Autodesk Inventor part; units mm, degrees
ref_plane "YZ Plane" through (0, 0, 0) normal (1, 0, 0) x (0, 1, 0)
ref_plane "XZ Plane" through (0, 0, 0) normal (0, 1, 0) x (-1, 0, 0)
ref_plane "XY Plane" through (0, 0, 0) normal (0, 0, 1) x (1, 0, 0)
sketch "Esquisse1" plane through (0, 0, 0) normal (0, 0, 1) x (1, 0, 0)
  line L0 (0, 0) -> (20, 0)
  line L1 (20, 0) -> (20, 20)
  line L2 (20, 20) -> (0, 20)
  line L3 (0, 20) -> (0, 0)
  circle A0 centre (10, 10) radius 2.15
  dimension "d0" = 20
  dimension "d1" = 20
  dimension "d2" = 4.3
extrude "Extrusion1" add sketch "Esquisse1" along normal blind 4
sketch "Esquisse2" plane through (0, 0, 4) normal (0, 0, 1) x (1, 0, 0)
  circle A0 centre (10, 10) radius 2.15
  line L0 (0, 20) -> (0, 0)
  circle A1 centre (10, 10) radius 2.15
  line L1 (0, 0) -> (20, 0)
  line L2 (20, 0) -> (20, 20)
  line L3 (20, 20) -> (0, 20)
  line L4 (0, 20) -> (0, 0)
  line L5 (13.4897, 12.0384) -> (13.5102, 7.997)
  line L6 (13.5102, 7.997) -> (10.0204, 5.9586)
  line L7 (10.0204, 5.9586) -> (6.5103, 7.9616)
  line L8 (6.5103, 7.9616) -> (6.4898, 12.003)
  line L9 (6.4898, 12.003) -> (6.4898, 20)
  line L10 (20, 20) -> (0, 20)
  line L11 (13.4897, 12.0384) -> (13.4897, 20)
  line L12 (6.4898, 20) -> (0, 20)
  line L13 (0, 0) -> (20, 0)
  line L14 (0, 0) -> (0, 20)
  line L15 (0, 0) -> (20, 0)
  line L16 (20, 0) -> (20, 20)
  line L17 (20, 20) -> (13.4897, 20)
  dimension "d5" = 7
  dimension "d6" = 0.29
extrude "Extrusion2" add sketch "Esquisse2" along normal blind 3.2 contours L3 L9 L8 L7 L6 L5 L11 L2 L1 L0
sketch "Esquisse3" plane through (0, 0, 7.2) normal (0, 0, 1) x (1, 0, 0)
  line L0 (6.4898, 20) -> (0, 20)
  line L1 (0, 20) -> (20, 20)
  line L2 (20, 20) -> (20, 0)
  line L3 (20, 0) -> (0, 0)
  line L4 (0, 0) -> (0, 20)
  circle A0 centre (10, 10) radius 2.15
  circle A1 centre (10, 10) radius 2.15
  point P0 (0, 0)
extrude "Extrusion4" add sketch "Esquisse3" along normal blind 4
sketch "Esquisse4" plane through (0, 0, 11.2) normal (0, 0, 1) x (1, 0, 0)
  line L0 (0, 20) -> (0, 0)
  line L1 (0, 10) -> (0, 0)
  line L2 (0, 0) -> (20, 0)
  line L3 (20, 0) -> (20, 10)
  line L4 (20, 0) -> (20, 20)
  line L5 (10, 10) -> (2.5, 10) construction
  line L6 (2.5, 10) -> (17.5, 10) construction
  arc A0 (2.5, 10) -> (17.5, 10) centre (10, 10) ccw
  arc A1 (17.5, 10) -> (2.5, 10) centre (10, 10) ccw
  line L7 (0, 10) -> (0, 20)
  line L8 (20, 20) -> (0, 20)
  line L9 (0, 20) -> (20, 20)
  line L10 (20, 20) -> (20, 10)
  line L11 (0, 10) -> (1.5, 10)
  line L12 (18.5, 10) -> (20, 10)
  arc A2 (18.5, 10) -> (1.5, 10) centre (10, 10) ccw
  dimension "d15" = 7.5
  dimension "d16" = 1
extrude "Extrusion5" add sketch "Esquisse4" along normal blind 20 contours L11 A2 L12 L3 L2 L0
sketch "Esquisse5" plane through (0, 0, 31.2) normal (0, 0, 1) x (1, 0, 0)
  circle A0 centre (10, 10) radius 7.5
  line L0 (0, 0) -> (20, 0)
  line L1 (20, 0) -> (20, 10)
  line L2 (20, 10) -> (18.5, 10)
  arc A1 (18.5, 10) -> (1.5, 10) centre (10, 10) ccw
  line L3 (1.5, 10) -> (0, 10)
  line L4 (0, 10) -> (0, 0)
  arc A2 (18.5, 10) -> (1.5, 10) centre (10, 10) ccw
  line L5 (6.0494, 17.5262) -> (6.0494, 16.3752)
  line L6 (13.9506, 16.3752) -> (13.9506, 17.5262)
  arc A3 (18.5, 10) -> (1.5, 10) centre (10, 10) ccw
  circle A4 centre (10, 10) radius 7.5
extrude "Extrusion6" add sketch "Esquisse5" along normal blind 78.5 contours A0 L6 A1 L2 L1 L0 L4 L3 L5
sketch "Esquisse6" plane through (0, 0, 109.7) normal (0, 0, 1) x (1, 0, 0)
  arc A0 (6.0494, 16.3752) -> (13.9506, 16.3752) centre (10, 10) ccw
  line L0 (0, 0) -> (20, 0)
  line L1 (11, 0.567) -> (11, 2.567)
  line L2 (9, 0.567) -> (9, 2.567)
  arc A1 (9, 2.567) -> (11, 2.567) centre (10, 10) ccw
  line L3 (9, 0.567) -> (11, 0.567)
  dimension "d23" = 2
  dimension "d24" = 2
extrude "Extrusion7" cut sketch "Esquisse6" against normal blind 90
sketch "Esquisse7" plane through (0, 0, 0) normal (-1, 0, 0) x (0, 0, 1)
  point P0 (0, 0)
sketch "Esquisse8" plane through (0, 0, 0) normal (-1, 0, 0) x (0, 0, 1)
  line L0 (109.7, 0) -> (109.7, 10)
  line L1 (0, 0) -> (109.7, 0)
  line L2 (109.7, 0) -> (109.7, 5)
  line L3 (109.7, 5) -> (0, 5)
  line L4 (0, 5) -> (0, 0)
extrude "Extrusion8" add sketch "Esquisse8" along normal blind 10
sketch "Esquisse9" plane through (20, 0, 0) normal (1, 0, 0) x (0, 0, -1)
  line L0 (-109.7, 0) -> (-109.7, 10)
  line L1 (0, 0) -> (-109.7, 0)
  line L2 (-109.7, 0) -> (-109.7, 5)
  line L3 (-109.7, 5) -> (0, 5)
  line L4 (0, 5) -> (0, 0)
extrude "Extrusion9" add sketch "Esquisse9" along normal blind 10
sketch "Esquisse10" plane through (20, 5, 109.7) normal (0, 1, 0) x (1, 0, 0)
  line L0 (10.0235, 93.2538) -> (5.0235, 93.2538) construction
  line L1 (0, 98.5) -> (0, 0) construction
  line L2 (5.0235, 93.2538) -> (5.0235, 8.1061) construction
  circle A0 centre (5.0235, 93.2538) radius 2.15
  circle A1 centre (5.0235, 53.2538) radius 2.15
  circle A2 centre (5.0235, 13.2538) radius 2.15
  circle A3 centre (-24.9765, 93.2538) radius 2.15
  circle A4 centre (-24.9765, 53.2538) radius 2.15
  circle A5 centre (-24.9765, 13.2538) radius 2.15
  point P0 (-20, 109.7)
  dimension "d31" = 5
  dimension "d32" = 4.3
  dimension "d35" = 40
  dimension "d38" = 30
extrude "Extrusion10" cut sketch "Esquisse10" against normal blind 10
sketch "Esquisse11" plane through (0, 0, 109.7) normal (0, 0, 1) x (1, 0, 0)
  line L0 (9, 0.567) -> (9, 2.567)
  arc A0 (6.0494, 16.3752) -> (9, 2.567) centre (10, 10) ccw
  line L1 (6.0494, 16.3752) -> (6.0494, 17.5262)
  arc A1 (6.0494, 17.5262) -> (1.5, 10) centre (10, 10) ccw
  line L2 (1.5, 10) -> (0, 10)
  line L3 (0, 10) -> (0, 5)
  line L4 (0, 5) -> (-10, 5)
  line L5 (-10, 0) -> (-10, 5)
  line L6 (30, 0) -> (-10, 0)
  line L7 (30, 5) -> (30, 0)
  line L8 (20, 5) -> (30, 5)
  line L9 (20, 5) -> (20, 10)
  line L10 (20, 10) -> (18.5, 10)
  arc A2 (18.5, 10) -> (13.9506, 17.5262) centre (10, 10) ccw
  line L11 (13.9506, 17.5262) -> (13.9506, 16.3752)
  arc A3 (11, 2.567) -> (13.9506, 16.3752) centre (10, 10) ccw
  line L12 (11, 2.567) -> (11, 0.567)
  line L13 (11, 0.567) -> (9, 0.567)
  point P0 (0, 0)
ref_plane "Plan de construction1" through (17.5, 10, 11.2) normal (1, 0, 0) x (0, 1, 0)
ref_plane "Plan de construction2" through (20, 20, 11.2) normal (1, 0, 0) x (0, 0, -1)
properties part number "lanceur"
Verification items for the finished model (mm, model axes). A direction names the side the tool comes from. Give positions to 0.01 mm unless a question says otherwise; leave off trailing zeros. Write each loop counter-clockwise with the first axis right and the second up, starting at its lowest first coordinate (ties: lowest second). Pieces come first, ordered by that corner, then holes.
(1) Cross-section at A-A (z = 25.5). Enter the section's corners in (x, y), plus the area to 3 significant figures.
(2) Cross-section at B-B (x = 24). Enter the section's corners in (y, z).
(3) Cross-section at C-C (z = 97.5). Enter the section's corners in (x, y), plus the area to 3 significant figures.
(4) Access from +Z, -Z, +X, -X, +Y, -Y to the whole of each face (thin tool, end or side, straight path). Record for faces 5 (the face through (6.49, 16, 6)), 6 (the face through (12, 8, 11.2)), 7 (the face through (0, 9, 42)).
(5) Mould release check, pull along X, two halves, no side actions. Record for faces 1 (the face through (10, 0.567, 65)), 2 (the face through (-6.56, 2.54, 14.99)), 3 (the face through (8, 2, 109.7)), 4 (the face through (-10, 3, 54)): +X half, -X half, draft (parallel to the pull), parting line (faces both ways), or undercut.
(6) Material ranges on line 1 (Z direction, x = 25, y = 4.5); line 2 (Z direction, x = 13, y = 16.25); line 3 (X direction, y = 10.25, z = 45), recorded low to high.
(7) Gauge pin test, flat ends, axial feed: pin 1 (3.5 mm diameter, centred on y = 14, z = 6.5, fed in from -X); pin 2 (6 mm diameter, centred on y = 13.5, z = 29, fed in from +X); pin 3 (0.9 mm diameter, centred on y = 17, z = 63.5, fed in from +X); pin 4 (5.5 mm diameter, centred on x = 10, y = 10, fed in from -Z). Record the tip position at first contact, or that the pin passes through.
Worked out:
1. outline: (-10, 0) - (30, 0) - (30, 5) - (20, 5) - (20, 10) - (18.5, 10) arc R8.5 ccw to (1.5, 10) - (0, 10) - (0, 5) - (-10, 5) - close; hole (9, 0.57) - (11, 0.57) - (11, 2.57) arc R7.5 ccw (long way) to (9, 2.57) - close
1. area: 233 mm2
2. outline: (0, 0) - (5, 0) - (5, 14.56) - (0, 14.56) - close; (0, 18.34) - (5, 18.34) - (5, 54.56) - (0, 54.56) - close; (0, 58.34) - (5, 58.34) - (5, 94.56) - (0, 94.56) - close; (0, 98.34) - (5, 98.34) - (5, 109.7) - (0, 109.7) - close
3. outline: (-10, 0) - (-6.85, 0) - (-6.85, 5) - (-10, 5) - close; (-3.1, 0) - (23.15, 0) - (23.15, 5) - (20, 5) - (20, 10) - (18.5, 10) arc R8.5 ccw to (13.95, 17.53) - (13.95, 16.38) arc R7.5 cw to (11, 2.57) - (11, 0.57) - (9, 0.57) - (9, 2.57) arc R7.5 cw to (6.05, 16.38) - (6.05, 17.53) arc R8.5 ccw to (1.5, 10) - (0, 10) - (0, 5) - (-3.1, 5) - close; (26.9, 0) - (30, 0) - (30, 5) - (26.9, 5) - close
3. area: 187 mm2
4. face 5: +Y
4. face 6: +Z
4. face 7: +Z, -Z, -X, +Y
5. face 1: undercut
5. face 2: undercut
5. face 3: draft
5. face 4: -X half
6. line 1: z = 0 to 14.3, 18.6 to 54.3, 58.6 to 94.3, 98.6 to 109.7
6. line 2: z = 0 to 4, 7.2 to 11.2
6. line 3: x = 1.5 to 2.5, 17.5 to 18.5
7. pin 1: stops at x = 0
7. pin 2: stops at x = 18.49
7. pin 3: stops at x = 15.42
7. pin 4: stops at z = 0
